```python
from build123d import *

# Parameters (mm, degrees)
SKETCH1_W               = 80
SKETCH1_H               = 80
BOSS_EXTRUDE1_DEPTH     = 16
CUT_EXTRUDE1_DEPTH      = 59.787753827
CUT_EXTRUDE1_DEPTH_BACK = 59.787753827
SKETCH2_R               = 1.75
SKETCH3_W               = 25
SKETCH3_H               = 16
CUT_EXTRUDE2_DEPTH      = 13
FILLET1_R               = 8
SKETCH4_W               = 16
SKETCH4_H               = 25
CUT_EXTRUDE3_DEPTH      = 3
BOSS_EXTRUDE2_DEPTH     = 23.5
CUT_EXTRUDE4_DEPTH      = 59.787753827
CUT_EXTRUDE4_DEPTH_BACK = 59.787753827
CUT_EXTRUDE5_DEPTH      = 59.787753827
CUT_EXTRUDE5_DEPTH_BACK = 59.787753827
SKETCH7_R               = 10
CUT_EXTRUDE6_DEPTH      = 59.787753827
CUT_EXTRUDE6_DEPTH_BACK = 59.787753827
CHAMFER1_SIZE           = 4
CHAMFER2_SIZE           = 30
BOSS_EXTRUDE4_START     = -3
SKETCH11_R              = 10
SKETCH11_R_2            = 4.25
BOSS_EXTRUDE4_DEPTH     = 3
SKETCH12_R              = 4
CUT_EXTRUDE7_DEPTH      = 5
CUT_EXTRUDE8_START      = -10
SKETCH13_R              = 3
SKETCH13_R_2            = 1.75
CUT_EXTRUDE8_DEPTH      = 10


with BuildPart() as part:
    # Sketch1 → Boss-Extrude1 (new body)
    with BuildSketch(Plane(origin=(0, 0, 0), x_dir=(1, 0, 0), z_dir=(0, 1, 0))):
        Rectangle(SKETCH1_W, SKETCH1_H)
    extrude(amount=-BOSS_EXTRUDE1_DEPTH)

    # Sketch2 → Cut-Extrude1 (cut, two sides: drawn at the far end of the back side and taken through both)
    with BuildSketch(Plane(origin=(0, 0, 0), x_dir=(1, 0, 0), z_dir=(0, 1, 0)).offset(-CUT_EXTRUDE1_DEPTH_BACK)):
        with Locations(Location((-11.5, -11.5, 0), (0, 0, 270))):
            Circle(SKETCH2_R)
        with Locations(Location((11.5, 11.5, 0), (0, 0, 270))):
            Circle(SKETCH2_R)
        with Locations(Location((22, 22, 0), (0, 0, 270))):
            Circle(SKETCH2_R)
        with Locations(Location((19, -34.5, 0), (0, 0, 270))):
            Circle(SKETCH2_R)
        with Locations(Location((34.5, -19, 0), (0, 0, 270))):
            Circle(SKETCH2_R)
        with Locations(Location((-34.5, 19, 0), (0, 0, 270))):
            Circle(SKETCH2_R)
        with Locations(Location((-19, 34.5, 0), (0, 0, 270))):
            Circle(SKETCH2_R)
    extrude(amount=CUT_EXTRUDE1_DEPTH + CUT_EXTRUDE1_DEPTH_BACK, mode=Mode.SUBTRACT)

    # Sketch3 → Cut-Extrude2 (cut)
    with BuildSketch(Plane(origin=(0, 0, 0), x_dir=(1, 0, 0), z_dir=(0, 1, 0))):
        with Locations((19, 0)):
            Rectangle(SKETCH3_W, SKETCH3_H)
        with Locations((-19, 0)):
            Rectangle(SKETCH3_W, SKETCH3_H)
    extrude(amount=-CUT_EXTRUDE2_DEPTH, mode=Mode.SUBTRACT)

    # Fillet1
    fillet1_edges = [part.edges().sort_by_distance(p)[0] for p in [
        (19, -13, 8),
        (19, -13, -8),
        (-19, -13, 8),
        (-19, -13, -8),
    ]]
    fillet(fillet1_edges, radius=FILLET1_R - 0.0001)  # a hair under: the kernel refuses the full size

    # Sketch4 → Cut-Extrude3 (cut)
    with BuildSketch(Plane(origin=(0, 0, 0), x_dir=(1, 0, 0), z_dir=(0, 1, 0))):
        with Locations((0, -19)):
            Rectangle(SKETCH4_W, SKETCH4_H)
        with Locations((0, 19)):
            Rectangle(SKETCH4_W, SKETCH4_H)
    extrude(amount=-CUT_EXTRUDE3_DEPTH, mode=Mode.SUBTRACT)

    # Sketch5 → Boss-Extrude2 (add)
    with BuildSketch(Plane(origin=(0, 0, 31.5), x_dir=(-1, 0, 0), z_dir=(0, 0, -1))):
        with BuildLine():
            ThreePointArc((1.5e-08, -3), (-3.464101608, -2.211102554), (-6.244997998, 0))
            Line((-6.244997998, 0), (-8, 0))
            Line((-8, 0), (-8, -3))
            Line((-8, -3), (1.5e-08, -3))
        make_face()
        with BuildLine():
            Line((8, -3), (8, 0))
            Line((8, 0), (6.244997998, 0))
            ThreePointArc((6.244997998, 0), (3.464101622, -2.211102548), (1.5e-08, -3))
            Line((1.5e-08, -3), (8, -3))
        make_face()
    boss_extrude2 = extrude(amount=BOSS_EXTRUDE2_DEPTH)

    # Mirror1: Boss-Extrude2 across plane
    add(boss_extrude2.mirror(Plane.XY))

    # Sketch6 → Cut-Extrude4 (cut, two sides: drawn at the far end of the back side and taken through both)
    with BuildSketch(Plane(origin=(0, 0, 0), x_dir=(0, 0, -1), z_dir=(1, 0, 0)).offset(-CUT_EXTRUDE4_DEPTH_BACK)):
        with BuildLine():
            ThreePointArc((-5, -5), (0, -10), (5, -5))
            Line((5, -5), (-5, -5))
        make_face()
        with BuildLine():
            Line((-5, -5), (5, -5))
            ThreePointArc((5, -5), (3.535533906, -1.464466094), (0, 0))
            ThreePointArc((0, 0), (-3.535533906, -1.464466094), (-5, -5))
        make_face()
        with BuildLine():
            Line((-5, 0), (-5, -5))
            ThreePointArc((-5, -5), (-3.535533906, -1.464466094), (0, 0))
            Line((0, 0), (-5, 0))
        make_face()
        with BuildLine():
            ThreePointArc((0, 0), (3.535533906, -1.464466094), (5, -5))
            Line((5, -5), (5, 0))
            Line((5, 0), (0, 0))
        make_face()
    extrude(amount=CUT_EXTRUDE4_DEPTH + CUT_EXTRUDE4_DEPTH_BACK, mode=Mode.SUBTRACT)

    # Sketch7 → Cut-Extrude5 (cut, two sides: drawn at the far end of the back side and taken through both)
    with BuildSketch(Plane(origin=(0, 0, 0), x_dir=(1, 0, 0), z_dir=(0, 1, 0)).offset(-CUT_EXTRUDE5_DEPTH_BACK)):
        with Locations(Location((19, -19, 0), (0, 0, 270))):
            Circle(SKETCH7_R)
        with Locations(Location((-19, 19, 0), (0, 0, 270))):
            Circle(SKETCH7_R)
    extrude(amount=CUT_EXTRUDE5_DEPTH + CUT_EXTRUDE5_DEPTH_BACK, mode=Mode.SUBTRACT)

    # Sketch9 → Cut-Extrude6 (cut, two sides: drawn at the far end of the back side and taken through both)
    with BuildSketch(Plane(origin=(0, 0, 0), x_dir=(1, 0, 0), z_dir=(0, 1, 0)).offset(-CUT_EXTRUDE6_DEPTH_BACK)):
        Polygon((-10, -18), (-18, -10), (-18, -18), align=None)
        Polygon((-10, -40), (-10, -18), (-18, -18), (-18, -10), (-40, -10), (-40, -40), align=None)
    extrude(amount=CUT_EXTRUDE6_DEPTH + CUT_EXTRUDE6_DEPTH_BACK, mode=Mode.SUBTRACT)

    # Chamfer1
    chamfer1_edges = [part.edges().sort_by_distance(p)[0] for p in [
        (-10, -8, 40),
        (-40, -8, 10),
        (40, -8, 40),
        (-40, -8, -40),
    ]]
    chamfer(chamfer1_edges, length=CHAMFER1_SIZE)

    # Chamfer2
    chamfer2_edges = [part.edges().sort_by_distance(p)[0] for p in [
        (40, -8, -40),
    ]]
    chamfer(chamfer2_edges, length=CHAMFER2_SIZE)

    # Sketch11 → Boss-Extrude4 (add)
    # profile 1 of 2: a face of its own
    with BuildSketch(Plane.XZ.offset(16).offset(BOSS_EXTRUDE4_START)):
        with Locations(Location((-19, -19, 0), (0, 0, 270))):
            Circle(SKETCH11_R)
        with Locations(Location((-19, -19, 0), (0, 0, 270))):
            Circle(SKETCH11_R_2, mode=Mode.SUBTRACT)
    # profile 2 of 2: a face of its own
    with BuildSketch(Plane.XZ.offset(16).offset(BOSS_EXTRUDE4_START)):
        with Locations(Location((19, 19, 0), (0, 0, 270))):
            Circle(SKETCH11_R)
        with Locations(Location((19, 19, 0), (0, 0, 270))):
            Circle(SKETCH11_R_2, mode=Mode.SUBTRACT)
    extrude(amount=BOSS_EXTRUDE4_DEPTH)

    # Sketch12 → Cut-Extrude7 (cut)
    with BuildSketch(Plane.XZ.offset(16)):
        with Locations(Location((0, 0, 0), (0, 0, 270))):
            Circle(SKETCH12_R)
        with Locations(Location((16.75, -16.75, 0), (0, 0, 270))):
            Circle(SKETCH12_R)
    extrude(amount=-CUT_EXTRUDE7_DEPTH, mode=Mode.SUBTRACT)

    # Sketch13 → Cut-Extrude8 (cut)
    # profile 1 of 7: a face of its own
    with BuildSketch(Plane.XZ.offset(16).offset(CUT_EXTRUDE8_START)):
        with Locations(Location((19, 34.5, 0), (0, 0, 270))):
            Circle(SKETCH13_R)
        with Locations(Location((19, 34.5, 0), (0, 0, 270))):
            Circle(SKETCH13_R_2, mode=Mode.SUBTRACT)
    # profile 2 of 7: a face of its own
    with BuildSketch(Plane.XZ.offset(16).offset(CUT_EXTRUDE8_START)):
        with Locations(Location((34.5, 19, 0), (0, 0, 270))):
            Circle(SKETCH13_R)
        with Locations(Location((34.5, 19, 0), (0, 0, 270))):
            Circle(SKETCH13_R_2, mode=Mode.SUBTRACT)
    # profile 3 of 7: a face of its own
    with BuildSketch(Plane.XZ.offset(16).offset(CUT_EXTRUDE8_START)):
        with Locations(Location((-11.5, 11.5, 0), (0, 0, 270))):
            Circle(SKETCH13_R)
        with Locations(Location((-11.5, 11.5, 0), (0, 0, 270))):
            Circle(SKETCH13_R_2, mode=Mode.SUBTRACT)
    # profile 4 of 7: a face of its own
    with BuildSketch(Plane.XZ.offset(16).offset(CUT_EXTRUDE8_START)):
        with Locations(Location((-34.5, -19, 0), (0, 0, 270))):
            Circle(SKETCH13_R)
        with Locations(Location((-34.5, -19, 0), (0, 0, 270))):
            Circle(SKETCH13_R_2, mode=Mode.SUBTRACT)
    # profile 5 of 7: a face of its own
    with BuildSketch(Plane.XZ.offset(16).offset(CUT_EXTRUDE8_START)):
        with Locations(Location((-19, -34.5, 0), (0, 0, 270))):
            Circle(SKETCH13_R)
        with Locations(Location((-19, -34.5, 0), (0, 0, 270))):
            Circle(SKETCH13_R_2, mode=Mode.SUBTRACT)
    # profile 6 of 7: a face of its own
    with BuildSketch(Plane.XZ.offset(16).offset(CUT_EXTRUDE8_START)):
        with Locations(Location((11.5, -11.5, 0), (0, 0, 270))):
            Circle(SKETCH13_R)
        with Locations(Location((11.5, -11.5, 0), (0, 0, 270))):
            Circle(SKETCH13_R_2, mode=Mode.SUBTRACT)
    # profile 7 of 7: a face of its own
    with BuildSketch(Plane.XZ.offset(16).offset(CUT_EXTRUDE8_START)):
        with Locations(Location((22, -22, 0), (0, 0, 270))):
            Circle(SKETCH13_R)
        with Locations(Location((22, -22, 0), (0, 0, 270))):
            Circle(SKETCH13_R_2, mode=Mode.SUBTRACT)
    extrude(amount=CUT_EXTRUDE8_DEPTH, mode=Mode.SUBTRACT)


solid = part.part
```
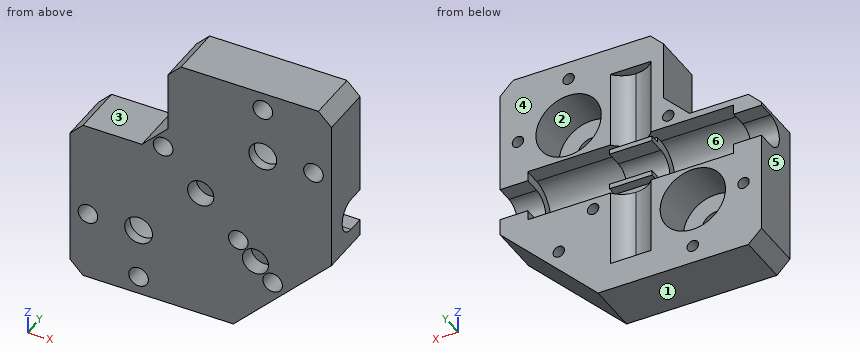
Work out the finished part from the listing and answer in its coordinate system (mm). Face numbers are marked on the shaded views. A direction names the side the tool comes from. Give positions to 0.01 mm unless a question says otherwise; leave off trailing zeros. Loops run counter-clockwise (first coordinate to the right, second up) from the corner with the lowest first, then second, coordinate; pieces in that order, holes last. Notation, with made-up numbers: (63.25, 10.5) -> (81.25, 10.5) arc R28 cw to (81.25, 28.5) -> close; hole circle Ø8 at (63.25, -38). An arc over 180 degrees is marked (long way). Write item = value, one per line. Start each with the question number.
(1) Given pin 1 Ø5 at (y, z) = (-11.5, 28.5) entering from -X; pin 2 Ø1.5 at (x, z) = (23, 4.5) entering from +Y; pin 3 Ø6 at (y, z) = (-5, 16) entering from -X, each flat-ended and moving along its own axis, determine where each tip first touches the part or whether it passes through.
(2) Find section C-C on z = 34.5. Give the vertices of the cut face in (x, y).
(3) Which of the six approach directions +Z, -Z, +X, -X, +Y, -Y give full straight-line access (tool end or side, diameter ignored) to the marked faces 1, 2 and 3?
(4) The mould has two halves that part along X. Classify the marked faces 4, 5 and 6: +X half, -X half, draft (parallel to the pull), parting line (faces both ways), or undercut.
(5) Find the intervals of material crossed by probe 1 along X at (y, z) = (-13.65, 19); probe 2 along X at (y, z) = (-13.4, -16.75); probe 3 along Z at (x, y) = (22.5, -5.5), in increasing order. Write a range as from..to.
(6) Find section A-A on y = -14.25. Give the number of separate pieces and of enclosed holes in the cut face, and give its area (3 significant figures).
(7) Find section D-D on z = 25. Give the vertices of the cut face in (x, y) (3 decimals).
From the geometry:
q1.pin_1 = -10
q1.pin_2 = -11.04
q1.pin_3 = -15
q2.outline = (-10, -16) -> (16, -16) -> (16, -6) -> (17.25, -6) -> (17.25, 0) -> (-10, 0) -> close; (20.75, -6) -> (22, -6) -> (22, -16) -> (40, -16) -> (40, 0) -> (20.75, 0) -> close
q3.face_1 = -Z, +X, -X, +Y, -Y
q3.face_2 = +Y
q3.face_3 = +Z, -X, +Y, -Y
q4.face_4 = draft
q4.face_5 = -X half
q4.face_6 = undercut
q5.probe_1 = -10..14.75, 23.25..31.5, 37.5..40
q5.probe_2 = -40..-36.48, -32.52..-22.61, -15.39..12.75, 20.75..33.25
q5.probe_3 = -27.5..-23.68, -20.32..-7.98, 7.98..9.63, 28.37..40
q6.separate_pieces = 1
q6.enclosed_holes = 11
q6.area = 4,640 mm^2
q7.outline = (-10, -16) -> (40, -16) -> (40, 0) -> (27, 0) -> (27, -13) -> (11, -13) -> (11, 0) -> (6.245, 0) arc R8 cw to (-6.245, 0) -> (-10, 0) -> close
